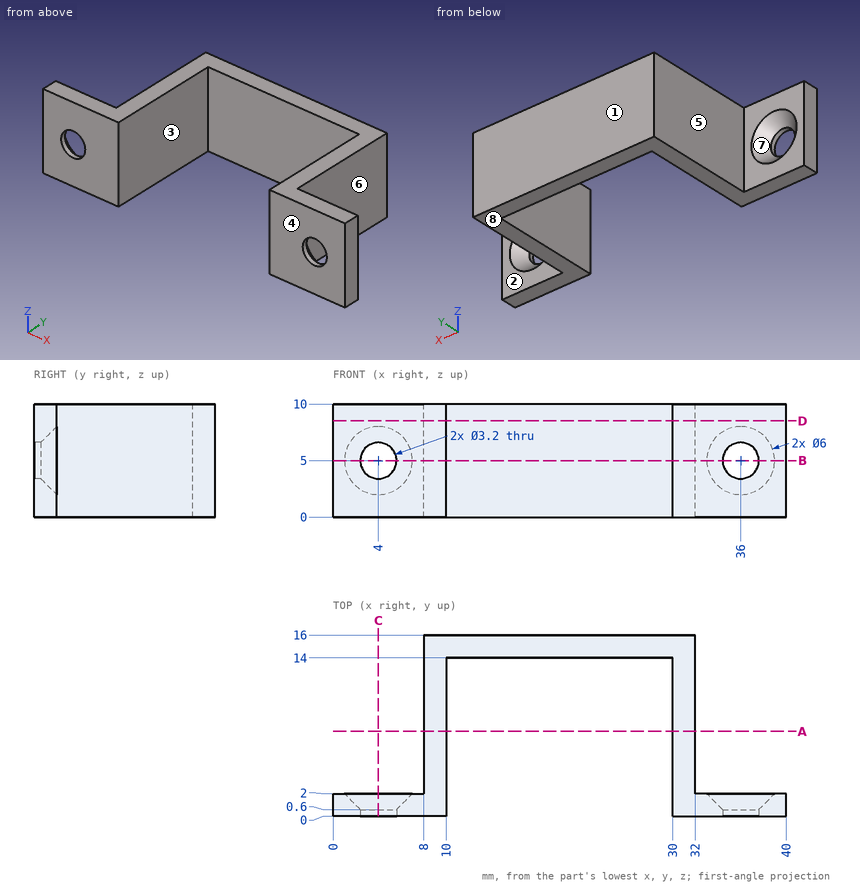
Here's the drawing with two shaded views (mm, measured from the low corner). I have some questions. A direction names the side the tool comes from. Give positions to 0.01 mm unless a question says otherwise; leave off trailing zeros. Order: outer loops, then holes, each group sorted by start corner. A loop starts at its lowest first (then second) coordinate and runs counter-clockwise, first axis right, second up. Notation, with made-up numbers: (-4.5, 74) -> (10.5, 74) arc R21 cw to (10.5, 106) -> close; hole circle Ø7 at (-26, -4.75). An arc over 180 degrees is marked (long way). One line per item, written item: value. Start each with the question number.
1. Imagine slicing it at A-A, the plane y = 7.5. List the corners of the cut face in (x, z) for me.
2. Imagine slicing it at D-D, the plane z = 8.5. List the corners of the cut face in (x, y) for me, plus the area to 3 significant figures.
3. For the marked faces 1, 2, 3, 4 and 5, which set-ups out of +Z, -Z, +X, -X, +Y, -Y let a thin tool reach every point of the face, with its end or its side?
4. Imagine slicing it at C-C, the plane x = 4. List the corners of the cut face in (y, z) for me, plus the area to 3 significant figures.
5. Imagine slicing it at B-B, the plane z = 5. List the corners of the cut face in (x, y) for me.
6. Will these pins go through, and if not, where does the flat tip stop? pin 1 Ø2 at (y, z) = (6, 8.5) entering from +X; pin 2 Ø2 at (x, z) = (12.5, 3) entering from -Y; pin 3 Ø2 at (y, z) = (7, 4) entering from -X; pin 4 Ø1.9 at (x, z) = (4, 5) entering from -Y.
7. I need wall thicknesses on probe 1 along X at (y, z) = (0.4, 5); probe 2 along X at (y, z) = (4.5, 1.75); probe 3 along Z at (x, y) = (4, 0.3). Which ranges of each line are inside material? Lowest first, please. Write a range as from..to.
8. We'd pull the mould along X, two halves only. Please class the marked faces 6, 7 and 8: released by +X, released by -X, zero draft, split by the parting line, or undercut.
Values follow:
1. outline: (8, 0) -> (10, 0) -> (10, 10) -> (8, 10) -> close; (30, 0) -> (32, 0) -> (32, 10) -> (30, 10) -> close
2. outline: (0, 0) -> (10, 0) -> (10, 14) -> (30, 14) -> (30, 0) -> (40, 0) -> (40, 2) -> (32, 2) -> (32, 16) -> (8, 16) -> (8, 2) -> (0, 2) -> close
2. area: 136 mm2
3. face 1: +Z, -Z, +X, -X, +Y
3. face 2: +Z, -Z, +X, +Y
3. face 3: +Z, -Z, -Y
3. face 4: +Z, -Z, +X, -X, -Y
3. face 5: +Z, -Z, -X, +Y
4. outline: (0, 0) -> (2, 0) -> (2, 2) -> (0.6, 3.4) -> (0, 3.4) -> close; (0, 6.6) -> (0.6, 6.6) -> (2, 8) -> (2, 10) -> (0, 10) -> close
4. area: 11.6 mm2
5. outline: (0, 0) -> (2.4, 0) -> (2.4, 0.6) -> (1, 2) -> (0, 2) -> close; (5.6, 0) -> (10, 0) -> (10, 14) -> (30, 14) -> (30, 0) -> (34.4, 0) -> (34.4, 0.6) -> (33, 2) -> (32, 2) -> (32, 16) -> (8, 16) -> (8, 2) -> (7, 2) -> (5.6, 0.6) -> close; (37.6, 0) -> (40, 0) -> (40, 2) -> (39, 2) -> (37.6, 0.6) -> close
6. pin 1: stops at x = 32
6. pin 2: stops at y = 14
6. pin 3: stops at x = 8
6. pin 4: passes through
7. probe 1: x = 0..2.4, 5.6..10, 30..34.4, 37.6..40
7. probe 2: x = 8..10, 30..32
7. probe 3: z = 0..3.4, 6.6..10
8. face 6: released by +X
8. face 7: undercut
8. face 8: zero draft
